The listing builds one solid part. Answer for the finished solid, in the listing's coordinates (mm). A direction names the side the tool comes from. Round coordinates to 2 decimals unless told otherwise and drop trailing zeros. Loops run counter-clockwise (first coordinate to the right, second up) from the corner with the lowest first, then second, coordinate; pieces in that order, holes last. Notation, with made-up numbers: (-12, 73) -> (42, 73) arc R7 ccw to (42, 82) -> close; hole circle Ø10 at (78, 59.5). An arc over 180 degrees is marked (long way). Use a Markdown table: item, result. Add a question column.
Q1. Section C-C on y = -29 is taken. Give the vertices of the cut face in (x, z), then the cut area to 3 significant figures.
Q2. For a pull along Z with two mould halves and no side action, classify faces 3 (the cylindrical face through (-14.287, -15.175, 14.248)), 4 (the flat face through (0, -15, -15)), 5 (the cylindrical face through (-1.08, -30.42, -4.88)), 6 (the cylindrical face through (-14.287, -0.752, 0.175)) as released by +Z, released by -Z, zero draft, split by the parting line, or undercut.
Q3. Which of the six approach directions +Z, -Z, +X, -X, +Y, -Y give full straight-line access (tool end or side, diameter ignored) to faces 1 (the flat face through (0, 0, 6)), 2 (the flat face through (-9, -30, 6))?
Q4. Given pin 1 Ø3 at (y, z) = (-39.5, 3) entering from -X; pin 2 Ø4 at (y, z) = (-53.5, -7) entering from -X; pin 3 Ø5 at (x, y) = (1.5, -41.5) entering from -Z, each flat-ended and moving along its own axis, determine where each tip first touches the part or whether it passes through.
Q5. Consider line 1 (Z direction, x = 0.25, y = -47.5); line 2 (Z direction, x = 0, y = -26); line 3 (Y direction, x = -0.5, z = -12.25). Determine where each line is inside the solid, lowest interval first.
Q6. Section D-D on z = -11 is taken. Give the vertices of the cut face in (x, y), then the cut area to 3 significant figures.
Q7. Section B-B on x = 0 is taken. Give the vertices of the cut face in (y, z).
Q8. Section A-A on z = 0 is taken. Give the vertices of the cut face in (x, y), then the cut area to 3 significant figures.
from build123d import *

# Parameters (mm, degrees)
F0_W     = 30
F0_H     = 30
F1_DEPTH = 30
F2_R     = 10
F3_DEPTH = 30
F4_R     = 2.5
F5_R     = 5
F6_DEPTH = 60.001


with BuildPart() as f1:
    # F0 (on Front) → F1 (new body)
    with BuildSketch(Plane.XZ):
        Rectangle(F0_W, F0_H)
    extrude(amount=F1_DEPTH)

    # F2 (on face) → F3 (join)
    with BuildSketch(Plane.XZ.offset(30)):
        Circle(F2_R)
    extrude(amount=F3_DEPTH)

    # F4
    f4_edges = [f1.edges().sort_by_distance(p)[0] for p in [
        (0, -30, 15),
        (-15, -30, 0),
        (0, -30, -15),
        (15, -30, 0),
        (-10, -60, 0),
        (-15, -15, 15),
        (-15, -15, -15),
        (-15, 0, 0),
        (15, -15, 15),
        (15, -15, -15),
        (15, 0, 0),
        (0, 0, 15),
        (0, 0, -15),
    ]]
    fillet(f4_edges, radius=F4_R)

    # F5 (on face) → F6 (cut, through all)
    with BuildSketch(Plane.XZ.offset(60)):
        Circle(F5_R)
    extrude(amount=-F6_DEPTH, mode=Mode.SUBTRACT)


solid = f1.part
Checked values:
| question | item | result |
|---|---|---|
| 1 | outline | (-14.5, -12.5) arc R2 ccw to (-12.5, -14.5) -> (12.5, -14.5) arc R2 ccw to (14.5, -12.5) -> (14.5, 12.5) arc R2 ccw to (12.5, 14.5) -> (-12.5, 14.5) arc R2 ccw to (-14.5, 12.5) -> close; hole circle Ø10 at (0, 0) |
| 1 | area | 759 mm2 |
| 2 | face 3 | released by +Z |
| 2 | face 4 | released by -Z |
| 2 | face 5 | undercut |
| 2 | face 6 | zero draft |
| 3 | face 1 | +Z, -Z, +X, -X, +Y |
| 3 | face 2 | -Y |
| 4 | pin 1 | stops at x = -9.89 |
| 4 | pin 2 | stops at x = -8.66 |
| 4 | pin 3 | stops at z = -10 |
| 5 | line 1 | z = -10 to -4.99, 4.99 to 10 |
| 5 | line 2 | z = -15 to -5, 5 to 15 |
| 5 | line 3 | y = -30 to 0 |
| 6 | outline | (-15, -27.5) arc R2.5 ccw to (-12.5, -30) -> (12.5, -30) arc R2.5 ccw to (15, -27.5) -> (15, -2.5) arc R2.5 ccw to (12.5, 0) -> (-12.5, 0) arc R2.5 ccw to (-15, -2.5) -> close |
| 6 | area | 895 mm2 |
| 7 | outline | (-60, -7.5) arc R2.5 ccw to (-57.5, -10) -> (-30, -10) -> (-30, -12.5) arc R2.5 ccw to (-27.5, -15) -> (-2.5, -15) arc R2.5 ccw to (0, -12.5) -> (0, -5) -> (-60, -5) -> close; (-60, 5) -> (0, 5) -> (0, 12.5) arc R2.5 ccw to (-2.5, 15) -> (-27.5, 15) arc R2.5 ccw to (-30, 12.5) -> (-30, 10) -> (-57.5, 10) arc R2.5 ccw to (-60, 7.5) -> close |
| 8 | outline | (-15, -27.5) arc R2.5 ccw to (-12.5, -30) -> (-10, -30) -> (-10, -57.5) arc R2.5 ccw to (-7.5, -60) -> (-5, -60) -> (-5, 0) -> (-12.5, 0) arc R2.5 ccw to (-15, -2.5) -> close; (5, -60) -> (7.5, -60) arc R2.5 ccw to (10, -57.5) -> (10, -30) -> (12.5, -30) arc R2.5 ccw to (15, -27.5) -> (15, -2.5) arc R2.5 ccw to (12.5, 0) -> (5, 0) -> close |
| 8 | area | 892 mm2 |
